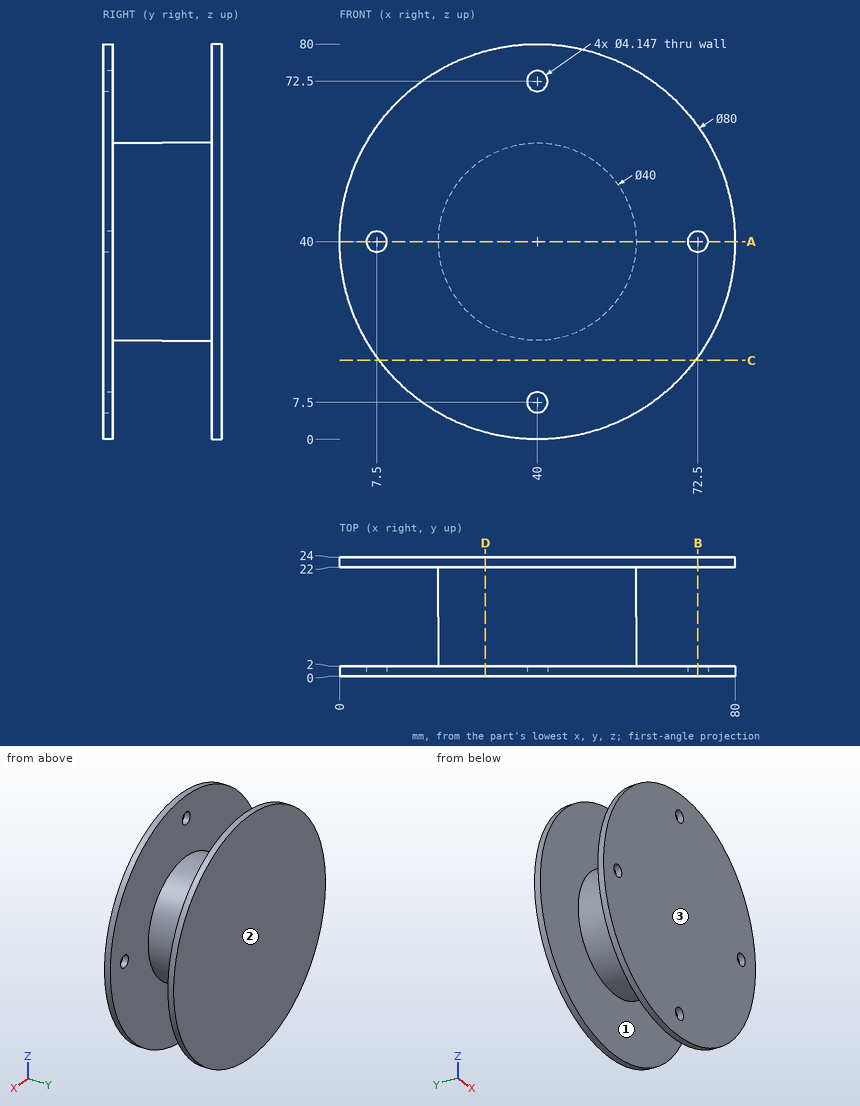
Geometry check sheet. Reference: drawing and pictorial views, mm from the part's lowest x, y, z. Give positions to 0.01 mm unless a question says otherwise; leave off trailing zeros. Loops run counter-clockwise (first coordinate to the right, second up) from the corner with the lowest first, then second, coordinate; pieces in that order, holes last. Notation, with made-up numbers: (-6.75, -33) - (1.25, -33) arc R31 cw to (1.25, -4) - close; hole circle Ø7 at (8.25, -21.5). An arc over 180 degrees is marked (long way). Use CSV: the item, a comma, the result in double quotes. Start each with the question number.
Q1. Section check A-A, the plane z = 40. Record the cut outline in (x, y).
Q2. Release check for a two-part mould opening along Y. For the marked faces 1, 2 and 3 record: +Y half, -Y half, draft (parallel to the pull), parting line (faces both ways), or undercut.
Q3. Scan lines: probe 1 along X at (y, z) = (1.05, 40); probe 2 along Y at (x, z) = (50.5, 63.5); probe 3 along X at (y, z) = (1.3, 72.5). Record each from-to range of solid material in increasing order. Write a range as from..to.
Q4. Section check B-B, the plane x = 72.5. Record the cut outline in (y, z), and give its area (3 significant figures).
Q5. Section check D-D, the plane x = 29.5. Record the cut outline in (y, z), and give its area (3 significant figures).
Q6. Go/stop test with flat-tipped pins: pin 1 Ø3 at (y, z) = (12.5, 32) entering from +X; pin 2 Ø1.5 at (x, y) = (21.5, 13) entering from +Z; pin 3 Ø12 at (y, z) = (4.5, 13.5) entering from -X; pin 4 Ø1.5 at (x, y) = (62.5, 6) entering from -Z. Record where each tip stops, or that it passes through.
Q7. Section check C-C, the plane z = 16. Record the cut outline in (x, y).
Findings below:
1,outline,"(0, 0) - (5.43, 0) - (5.43, 2) - (0, 2) - close; (0, 22) - (20, 22) - (20, 2) - (9.57, 2) - (9.57, 0) - (70.43, 0) - (70.43, 2) - (60, 2) - (60, 22) - (80, 22) - (80, 24) - (0, 24) - close; (74.57, 0) - (80, 0) - (80, 2) - (74.57, 2) - close"
2,face 1,"undercut"
2,face 2,"+Y half"
2,face 3,"-Y half"
3,probe 1,"x = 0..5.43, 9.57..70.43, 74.57..80"
3,probe 2,"y = 0..2, 22..24"
3,probe 3,"x = 16.68..37.93, 42.07..63.32"
4,outline,"(0, 16.68) - (2, 16.68) - (2, 37.93) - (0, 37.93) - close; (0, 42.07) - (2, 42.07) - (2, 63.32) - (0, 63.32) - close; (22, 16.68) - (24, 16.68) - (24, 63.32) - (22, 63.32) - close"
4,area,"178 mm^2"
5,outline,"(0, 1.4) - (2, 1.4) - (2, 22.98) - (22, 22.98) - (22, 1.4) - (24, 1.4) - (24, 78.6) - (22, 78.6) - (22, 57.02) - (2, 57.02) - (2, 78.6) - (0, 78.6) - close"
5,area,"990 mm^2"
6,pin 1,"stops at x = 58.91"
6,pin 2,"stops at z = 49.22"
6,pin 3,"stops at x = 5.98"
6,pin 4,"passes through"
7,outline,"(8, 0) - (72, 0) - (72, 2) - (8, 2) - close; (8, 22) - (72, 22) - (72, 24) - (8, 24) - close"
